Build history of the part. All positions in model axes, mm. Face numbers are marked on the shaded views. Round coordinates to 2 decimals unless told otherwise and drop trailing zeros. Loops run counter-clockwise (first coordinate to the right, second up) from the corner with the lowest first, then second, coordinate; pieces in that order, holes last.
from build123d import *

# Parameters (mm, degrees)
BOSS_EXTRUDE1_DEPTH = 26
SKETCH2_R           = 1.7
CUT_EXTRUDE1_DEPTH  = 31
CUT_EXTRUDE2_DEPTH  = 1


with BuildPart() as part:
    # Sketch1 → Boss-Extrude1 (new body)
    with BuildSketch(Plane(origin=(0, 0, 0), x_dir=(1, 0, 0), z_dir=(0, 1, 0))):
        with BuildLine():
            Line((-46.998275301, 32.528571429), (-46.998275301, -39.471428571))
            Line((-46.998275301, -39.471428571), (-16.998275301, -39.471428571))
            Line((-16.998275301, -39.471428571), (-16.998275301, -25.971428571))
            ThreePointArc((-16.998275301, -25.971428571), (-39.498275301, -3.471428571), (-16.998275301, 19.028571429))
            Line((-16.998275301, 19.028571429), (-16.998275301, 32.528571429))
            Line((-16.998275301, 32.528571429), (-46.998275301, 32.528571429))
        make_face()
    extrude(amount=BOSS_EXTRUDE1_DEPTH)

    # Sketch2 → Cut-Extrude1 (cut, through all)
    with BuildSketch(Plane(origin=(-16.998275301, 0, 0), x_dir=(0, 0, -1), z_dir=(1, 0, 0))):
        with Locations((-34.471428571, 13)):
            Circle(SKETCH2_R)
        with Locations((27.528571429, 13)):
            Circle(SKETCH2_R)
    extrude(amount=-CUT_EXTRUDE1_DEPTH, mode=Mode.SUBTRACT)

    # Sketch3 → Cut-Extrude2 (cut)
    with BuildSketch(Plane(origin=(-16.998275301, 0, 0), x_dir=(0, 0, -1), z_dir=(1, 0, 0))):
        Polygon((-34.164231178, 21.664809495), (-32.617436306, 21.664809495), (-32.617436306, 21.33916847), (-33.87929528, 21.33916847), (-33.87929528, 20.362245393), (-32.617436306, 20.362245393), (-32.617436306, 20.036604367), (-33.87929528, 20.036604367), (-33.87929528, 18.489809495), (-34.164231178, 18.489809495), align=None)
        Polygon((-31.657685705, 21.664809495), (-31.070641434, 21.664809495), (-31.070641434, 18.489809495), (-31.355577332, 18.489809495), (-31.355577332, 21.33916847), (-31.84403887, 21.33916847), align=None)
    extrude(amount=-CUT_EXTRUDE2_DEPTH, mode=Mode.SUBTRACT)


solid = part.part
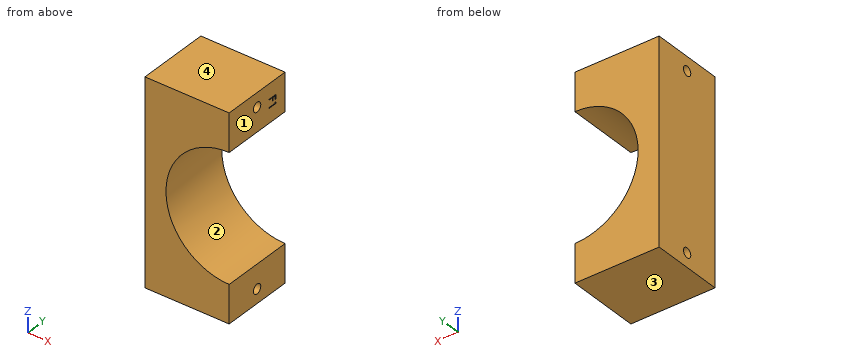
(1) Pull direction Z, two halves, no side cores. Call the marked faces 1, 2, 3 and 4: +Z half, -Z half, draft (parallel to the pull), parting line (faces both ways), or undercut.
Responses:
face 1: draft
face 2: undercut
face 3: -Z half
face 4: +Z half
(2) Probe line 1 (Y direction, x = -24.25, z = -27.5); line 2 (Z direction, x = -20.25, y = 8.25); line 3 (Z direction, x = -34.25, y = 24.5). List the from-to ranges inside material, lowest first.
Responses:
line 1: y = 0 to 11.3, 14.7 to 26
line 2: z = -32.53 to -18.79, 25.74 to 39.47
line 3: z = -32.53 to -10.97, 17.92 to 39.47
(3) Slice it at B-B on y = 13. List the corners of the cut face in (x, z), plus the area to 3 significant figures.
Responses:
outline: (-47, -32.53) - (-17, -32.53) - (-17, -29.23) - (-47, -29.23) - close; (-47, -25.83) - (-17, -25.83) - (-17, -19.03) arc R22.5 cw to (-17, 25.97) - (-17, 32.77) - (-47, 32.77) - close; (-47, 36.17) - (-17, 36.17) - (-17, 39.47) - (-47, 39.47) - close
area: 1,160 mm2
(4) Pin check, flat tips, straight feed: P1, Ø6, axis at y = 12, z = 5, coming from the +X side; P2, Ø5, axis at y = 12.5, z = -1.5, coming from the +X side; P3, Ø4, axis at y = 13, z = -27.53, coming from the -X side. Stop position of each tip, or through.
Responses:
P1: stops at x = -39.04
P2: stops at x = -38.22
P3: stops at x = -47
(5) Slice it at C-C on y = 17.25. List the corners of the cut face in (x, z), plus the area to 3 significant figures.
Responses:
outline: (-47, -32.53) - (-17, -32.53) - (-17, -19.03) arc R22.5 cw to (-17, 25.97) - (-17, 39.47) - (-47, 39.47) - close
area: 1,360 mm2
(6) Slice it at A-A on x = -26. List the corners of the cut face in (y, z), plus the area to 3 significant figures.
Responses:
outline: (0, -32.53) - (26, -32.53) - (26, -17.15) - (0, -17.15) - close; (0, 24.09) - (26, 24.09) - (26, 39.47) - (0, 39.47) - close; hole circle Ø3.4 at (13, -27.53); hole circle Ø3.4 at (13, 34.47)
area: 782 mm2
(7) Slice it at D-D on x = -38. List the corners of the cut face in (y, z), plus the area to 3 significant figures.
Responses:
outline: (0, -32.53) - (26, -32.53) - (26, -4.6) - (0, -4.6) - close; (0, 11.54) - (26, 11.54) - (26, 39.47) - (0, 39.47) - close; hole circle Ø3.4 at (13, -27.53); hole circle Ø3.4 at (13, 34.47)
area: 1,430 mm2
